from build123d import *

# Parameters (mm, degrees)
SKETCH1_R             = 30
SKETCH2_R             = 27.5
SKETCH3_R             = 25.85
BUTTON_DEPTH          = 3.25
SKETCH4_R             = 12
THREAD_DEPTH          = 29.4
SKETCH5_R             = 1.675
ALIGNMENT_STUDS_DEPTH = 3.7
SKETCH6_W             = 28
SKETCH6_H             = 17
BOSS_EXTRUDE1_DEPTH   = 10
SKETCH6_3_W           = 10
SKETCH6_3_H           = 1
BOSS_EXTRUDE2_DEPTH   = 3.25
BOSS_EXTRUDE3_DEPTH   = 3.25


with BuildPart() as part:
    # Sketch1 → Frame section 0
    with BuildSketch(Plane(origin=(0, 0, 0), x_dir=(1, 0, 0), z_dir=(0, 1, 0))):
        Circle(SKETCH1_R)
    # Sketch2 → Frame section 1
    with BuildSketch(Plane(origin=(0, 10.25, 0), x_dir=(1, 0, 0), z_dir=(0, 1, 0))):
        Circle(SKETCH2_R)
    loft()

    # Sketch3 → Button (add)
    with BuildSketch(Plane(origin=(0, 10.25, 0), x_dir=(1, 0, 0), z_dir=(0, 1, 0))):
        with Locations(Location((0, 0, 0), (0, 0, 90))):
            Circle(SKETCH3_R)
    extrude(amount=BUTTON_DEPTH)

    # Sketch4 → Thread (add)
    with BuildSketch(Plane.XZ):
        with Locations(Location((0, 0, 0), (0, 0, 270))):
            Circle(SKETCH4_R)
    extrude(amount=THREAD_DEPTH)

    # Sketch5 → Alignment studs (add)
    with BuildSketch(Plane.XZ):
        with Locations(Location((0, 18.75, 0), (0, 0, 90))):
            Circle(SKETCH5_R)
        with Locations(Location((0, -18.75, 0), (0, 0, 90))):
            Circle(SKETCH5_R)
    extrude(amount=ALIGNMENT_STUDS_DEPTH)

    # Sketch6 → Boss-Extrude1 (add, symmetric)
    with BuildSketch(Plane(origin=(0, 0, 0), x_dir=(0, 0, -1), z_dir=(1, 0, 0))):
        with Locations((0, -37.9)):
            Rectangle(SKETCH6_W, SKETCH6_H)
    extrude(amount=BOSS_EXTRUDE1_DEPTH, both=True)

    # Sketch6_3 → Boss-Extrude2 (add, symmetric)
    with BuildSketch(Plane(origin=(0, 0, 0), x_dir=(0, 0, -1), z_dir=(1, 0, 0))):
        Polygon((0.5, -50.4), (0.5, -46.4), (-0.5, -46.4), (-0.5, -49.4), (-9, -49.4), (-9, -50.4), align=None)
        with Locations((-19, -37.9)):
            Rectangle(SKETCH6_3_W, SKETCH6_3_H)
    extrude(amount=BOSS_EXTRUDE2_DEPTH, both=True)

    # Sketch7 → Boss-Extrude3 (add, symmetric)
    with BuildSketch(Plane.XY):
        Polygon((-10, -37.4), (-14, -37.4), (-14, -46.4), (-13, -46.4), (-13, -38.4), (-10, -38.4), align=None)
        Polygon((10, -37.4), (10, -38.4), (13, -38.4), (13, -46.4), (14, -46.4), (14, -37.4), align=None)
    extrude(amount=BOSS_EXTRUDE3_DEPTH, both=True)


solid = part.part
Check sheet for the modelled part. Datum: model origin and axes. Units: mm. A direction names the side the tool comes from. Coordinates: 2 decimals unless noted, no trailing zeros. Loops run counter-clockwise (first coordinate to the right, second up) from the corner with the lowest first, then second, coordinate; pieces in that order, holes last. Notation, with made-up numbers: (62, -13) -> (117, -13) arc R21 ccw to (117, -8) -> close; hole circle Ø9 at (85, 43). An arc over 180 degrees is marked (long way). Answer in a Markdown table with one row per item.
1. Release check for a two-part mould opening along Y. For faces 4 (the face through (0, -3.7, 19)), 5 (the face through (-21.92, 9.75, 16.81)), 6 (the face through (0, -38, -14)), 7 (the face through (0, -50.4, 4)) record: released by +Y, released by -Y, zero draft, split by the parting line, or undercut.
Check values:
| item | result |
|---|---|
| face 4 | undercut |
| face 5 | released by +Y |
| face 6 | zero draft |
| face 7 | released by -Y |
2. Go/stop test with flat-tipped pins: pin 1 (6 mm diameter, centred on x = 9.5, z = -23, fed in from -Y); pin 2 (13.5 mm diameter, centred on y = -41.5, z = -7, fed in from +X); pin 3 (1.1 mm diameter, centred on x = 0, y = -38, fed in from +Z). Record where each tip stops, or that it passes through.
Check values:
| item | result |
|---|---|
| pin 1 | stops at y = 0 |
| pin 2 | stops at x = 14 |
| pin 3 | stops at z = 24 |
3. Material ranges on line 1 along Y through (x, z) = (-2, 21.5); line 2 along Y through (x, z) = (15, 6); line 3 along Y through (x, z) = (-18, -20), recorded low to high. Write a range as [from, to].
Check values:
| item | result |
|---|---|
| line 1 | y = [-38.4, -37.4], [0, 13.5] |
| line 2 | y = [0, 13.5] |
| line 3 | y = [0, 10.25] |
4. Sectioned sample at B-B, the plane y = -1.5. Record the boundary of the cut face in (x, z) (3 decimals).
Check values:
| item | result |
|---|---|
| outline | circle Ø24 at (0, 0); circle Ø3.35 at (0, -18.75); circle Ø3.35 at (0, 18.75) |
5. Access from +Z, -Z, +X, -X, +Y, -Y to the whole of each face (thin tool, end or side, straight path). Record for faces 1 (the face through (15.729, 11.852, 20.514)), 2 (the face through (-14, -42, 0)), 3 (the face through (13, 0, 0)).
Check values:
| item | result |
|---|---|
| face 1 | +Y |
| face 2 | +Z, -Z, -X, -Y |
| face 3 | none |
